The listing builds one solid part. Answer for the finished solid, in the listing's coordinates (mm). A direction names the side the tool comes from. Round coordinates to 2 decimals unless told otherwise and drop trailing zeros. Write each loop counter-clockwise with the first axis right and the second up, starting at its lowest first coordinate (ties: lowest second). Pieces come first, ordered by that corner, then holes. Notation, with made-up numbers: (79, 82.5) -> (96, 82.5) arc R6 ccw to (96, 91.5) -> close; hole circle Ø3 at (-6, 89.25). An arc over 180 degrees is marked (long way). Write each question's results on one line, items separated by ' | '. Start each with the question number.
Autodesk Inventor part; units mm, degrees
ref_plane "YZ Plane" through (0, 0, 0) normal (1, 0, 0) x (0, 1, 0)
ref_plane "XZ Plane" through (0, 0, 0) normal (0, 1, 0) x (-1, 0, 0)
ref_plane "XY Plane" through (0, 0, 0) normal (0, 0, 1) x (1, 0, 0)
sketch "Sketch1" plane through (0, 0, 0) normal (0, 0, 1) x (1, 0, 0)
  line L0 (0, 25.4) -> (-28.702, 25.4) construction
  line L1 (0, 25.4) -> (-93.98, 25.4) construction
  line L2 (-93.98, 25.4) -> (-90.805, 25.4) construction
  line L3 (-90.805, 25.4) -> (-84.455, 22.4389) construction
  line L4 (-90.805, 25.4) -> (-90.805, 22.4389) construction
  line L5 (-90.805, 0) -> (-93.98, 0)
  line L6 (-28.702, 59.6457) -> (-28.702, -91.9304) construction
  arc A0 (-28.9184, -9.248) -> (-32.3684, -1.8494) centre (-35.052, -7.6045) ccw
  line L7 (-74.93, -180.9657) -> (-28.702, -8.4405)
  line L8 (-90.805, 25.4) -> (-90.805, 0)
  line L9 (-90.805, 25.4) -> (-32.3684, -1.8494)
  line L10 (-28.702, -7.6045) -> (-60.452, -7.6045) construction
  line L11 (-60.452, -126.9331) -> (-54.102, -126.9331) construction
  line L12 (-54.102, -126.9331) -> (-54.102, -103.2346) construction
  line L13 (-54.102, -103.2346) -> (-60.452, -103.2346)
  line L14 (-60.452, 11.2462) -> (-60.452, 1.7212) construction
  line L15 (-60.452, 11.2462) -> (-60.452, 4.7154) construction
  line L16 (-60.452, 4.7154) -> (-46.4468, 4.7154)
  line L17 (-93.98, 0) -> (-93.98, -12.7) construction
  line L18 (-60.452, -12.7) -> (-73.152, -12.7) construction
  line L19 (-93.98, -12.7) -> (-93.98, -25.4) construction
  line L20 (-93.98, -25.4) -> (-93.98, -88.9) construction
  line L21 (-93.98, -88.9) -> (-81.28, -88.9) construction
  line L22 (-81.28, -88.9) -> (-81.28, -25.4) construction
  line L23 (-93.98, -25.4) -> (-81.28, -25.4)
  line L24 (-81.28, -25.4) -> (-81.28, -88.9)
  line L25 (-81.28, -88.9) -> (-93.98, -88.9)
  line L26 (-93.98, -12.7) -> (-73.152, -12.7)
  line L27 (-73.152, -138.7824) -> (-63.627, -138.7824)
  line L28 (-81.28, -88.9) -> (-81.28, -180.9657)
  line L29 (-81.28, -180.9657) -> (-74.93, -180.9657)
  line L30 (-73.152, -12.7) -> (-73.152, -138.7824)
  line L31 (-87.63, -25.4) -> (-87.63, -31.3436)
  line L32 (-87.63, -31.3436) -> (-93.98, -31.3436)
  line L33 (-93.98, 0) -> (-93.98, -25.4)
  line L34 (-93.98, -31.3436) -> (-93.98, -88.9)
  line L35 (-28.9184, -9.248) -> (-84.2906, -215.9)
  line L36 (-84.2906, -215.9) -> (-87.4656, -215.9)
  line L37 (-66.802, -38.1) -> (-73.152, -38.1)
  line L38 (-66.802, -38.1) -> (-66.802, 4.7154)
  line L39 (-66.802, 4.7154) -> (-60.452, 4.7154)
  line L40 (-66.802, -38.1) -> (-60.452, -103.2346)
  line L41 (-60.452, 11.2462) -> (-60.452, 4.7154) construction
  line L42 (-60.452, -7.6045) -> (-60.452, -12.7) construction
  line L43 (-60.452, -103.2346) -> (-60.452, -126.9331) construction
  line L44 (0, -319.0244) -> (0, 122.7573)
  line L45 (0, -88.9) -> (-101.6, -88.9) construction
  line L46 (-101.6, -88.9) -> (-87.4656, -215.9)
  line L47 (-97.155, -88.9) -> (-97.155, -92.075)
  line L48 (-97.155, -92.075) -> (-93.98, -92.075)
  line L49 (-93.98, -92.075) -> (-93.98, -88.9)
  line L50 (-101.6, -88.9) -> (-97.155, -88.9)
  line L51 (-93.98, -88.9) -> (-81.28, -88.9)
  line L52 (-84.455, -88.9) -> (-84.455, -155.5657)
  line L53 (-84.455, -155.5657) -> (-81.28, -155.5657)
  point P0 (0, 0)
  point P1 (-93.98, -255.9127)
  point P2 (-88.7095, 22.4389)
  dimension "d0" = 28.702
  dimension "d1" = 93.98
  dimension "d2" = 3.175
  dimension "d3" = 25
  dimension "d5" = 25.4
  dimension "d6" = 25.4
  dimension "d8" = 12.7
  dimension "d12" = 31.75
  dimension "d13" = 6.35
  dimension "d16" = 12.7
  dimension "d17" = 12.7
  dimension "d18" = 12.7
  dimension "d19" = 63.5
  dimension "d20" = 12.7
  dimension "d22" = 9.525
  dimension "d23" = 6.35
  dimension "d25" = 5.9436
  dimension "d27" = 3.175
  dimension "d30" = 107.95
  dimension "d31" = 6.35
  dimension "d32" = 25.4
  dimension "d33" = 20.3552
  dimension "d34" = 15
  dimension "d36" = 101.6
  dimension "d37" = 127
  dimension "d38" = 3.175
  dimension "d39" = 3.175
  dimension "d42" = 3.175
  dimension "d43" = 25.4
revolve "Revolution2" add sketch "Sketch1" angle 360 about axis through (0, -10, 0) along (0, 1, 0) contours L35 L36 L46 L50 L47 L48 L49 L25 L52 L53 L28 L29
thread "Thread1"
properties part number "aluminum_skirt" material "Aluminum 6061"
Q1. The part is cut by section A-A, the plane x = 0. Write down the section's boundary in (y, z) (3 decimals).
Q2. The part is cut by section C-C, the plane y = -130. Write down the section's boundary in (x, z) (3 decimals).
Q3. The part is cut by section B-B, the plane z = 0. Write down the section's boundary in (x, y) (3 decimals).
Q4. The part is cut by section D-D, the plane y = -115. Write down the section's boundary in (x, z) (3 decimals), then the cut area to 3 significant figures.
Q5. Determine the mould class of faces 3 (the flat face through (77, -88.9, 35.2)), 4 (the cylindrical face through (10.58, -168.44, -80.59)), 5 (the conical face through (73.85, -165.62, -56.63)), 6 (the flat face through (51, -92.075, 80)) for opening direction Z: pulls with the +Z half, pulls with the -Z half, needs draft (parallel to the pull), parting line crosses it, or undercut.
Q6. Each of these flat-tipped pins is pushed along its axis until it touches: pin 1 (4 mm diameter, centred on y = -166.5, z = 51.5, fed in from -X); pin 2 (4 mm diameter, centred on x = 6, z = 75, fed in from +Y); pin 3 (8 mm diameter, centred on y = -133, z = -65, fed in from +X). Where does it stop, or does it pass through?
Q7. For faces 1 (the cylindrical face through (-38.971, -122.7, 74.926)), 2 (the flat face through (46, -215.9, 72)), determine the directions among +Z, -Z, +X, -X, +Y, -Y from which every point of the face is accessible in a straight line to the end or side of a thin tool.
Q8. Find the intervals of material crossed by line 1 (Z direction, x = 0, y = -90.75) (3 decimals); line 2 (Z direction, x = 56, y = -210.5); line 3 (X direction, y = -184, z = -51.5), in increasing order.
Answers follow:
1) outline: (-215.9, -87.466) -> (-88.9, -101.6) -> (-88.9, -97.155) -> (-92.075, -97.155) -> (-92.075, -93.98) -> (-88.9, -93.98) -> (-88.9, -84.455) -> (-155.566, -84.455) -> (-155.566, -81.28) -> (-180.966, -81.28) -> (-180.966, -74.93) -> (-215.9, -84.291) -> close; (-215.9, 84.291) -> (-180.966, 74.93) -> (-180.966, 81.28) -> (-155.566, 81.28) -> (-155.566, 84.455) -> (-88.9, 84.455) -> (-88.9, 93.98) -> (-92.075, 93.98) -> (-92.075, 97.155) -> (-88.9, 97.155) -> (-88.9, 101.6) -> (-215.9, 87.466) -> close
2) outline: circle Ø194.052 at (0, 0); hole circle Ø168.91 at (0, 0)
3) outline: (-101.6, -88.9) -> (-87.466, -215.9) -> (-84.291, -215.9) -> (-74.93, -180.966) -> (-81.28, -180.966) -> (-81.28, -155.566) -> (-84.455, -155.566) -> (-84.455, -88.9) -> (-93.98, -88.9) -> (-93.98, -92.075) -> (-97.155, -92.075) -> (-97.155, -88.9) -> close; (74.93, -180.966) -> (84.291, -215.9) -> (87.466, -215.9) -> (101.6, -88.9) -> (97.155, -88.9) -> (97.155, -92.075) -> (93.98, -92.075) -> (93.98, -88.9) -> (84.455, -88.9) -> (84.455, -155.566) -> (81.28, -155.566) -> (81.28, -180.966) -> close
4) outline: circle Ø197.39 at (0, 0); hole circle Ø168.91 at (0, 0) | area: 8,190 mm^2
5) face 3: needs draft | face 4: undercut | face 5: parting line crosses it | face 6: undercut
6) pin 1: x = -78.72 | pin 2: y = -180.97 | pin 3: x = 75.07
7) face 1: +Y | face 2: +Z, -Z, +X, -X, -Y
8) line 1: -101.394 to -97.155, -93.98 to -84.455, 84.455 to 93.98, 97.155 to 101.394 | line 2: -67.97 to -61.05, 61.05 to 67.97 | line 3: -75.04 to -55.54, 55.54 to 75.04
